The listing builds one solid part. Answer for the finished solid, in the listing's coordinates (mm). A direction names the side the tool comes from. Round coordinates to 2 decimals unless told otherwise and drop trailing zeros. Loops run counter-clockwise (first coordinate to the right, second up) from the corner with the lowest first, then second, coordinate; pieces in that order, holes last. Notation, with made-up numbers: (63, 29) - (100, 29) arc R25 ccw to (100, 62) - close; hole circle Ø4 at (14.5, -13.5). An arc over 180 degrees is marked (long way). One line per item, written item: value.
```python
from build123d import *

# Parameters (mm, degrees)
SKETCH_W        = 92
SKETCH_H        = 130
PAD_DEPTH       = 44
SKETCH001_W     = 88
SKETCH001_H     = 126
POCKET_DEPTH    = 40
SKETCH002_W     = 87.518665
SKETCH002_H     = 101
POCKET001_DEPTH = 2
SKETCH004_W     = 80
SKETCH004_H     = 80
POCKET003_DEPTH = 2
SKETCH005_W     = 88
SKETCH005_H     = 40
POCKET004_DEPTH = 2


with BuildPart() as part:
    # Sketch → Pad (new body)
    with BuildSketch(Plane.XY):
        Rectangle(SKETCH_W, SKETCH_H)
    extrude(amount=PAD_DEPTH)

    # Sketch001 → Pocket (cut)
    with BuildSketch(Plane.XY.offset(42)):
        Rectangle(SKETCH001_W, SKETCH001_H)
    extrude(amount=-POCKET_DEPTH, mode=Mode.SUBTRACT)

    # Sketch002 → Pocket001 (cut)
    with BuildSketch(Plane.XY.offset(44)):
        with Locations((0.240668, -2.5)):
            Rectangle(SKETCH002_W, SKETCH002_H)
    extrude(amount=-POCKET001_DEPTH, mode=Mode.SUBTRACT)

    # Sketch004 → Pocket003 (cut)
    with BuildSketch(Plane.XY):
        with Locations((0, -2)):
            Rectangle(SKETCH004_W, SKETCH004_H)
    extrude(amount=POCKET003_DEPTH, mode=Mode.SUBTRACT)

    # Sketch005 → Pocket004 (cut)
    with BuildSketch(Plane.XZ.offset(-65)):
        with Locations((0, 22)):
            Rectangle(SKETCH005_W, SKETCH005_H)
    extrude(amount=POCKET004_DEPTH, mode=Mode.SUBTRACT)


solid = part.part
```
1) Consider L1, parallel to X at y = -23, z = 33.5; L2, parallel to Z at x = -2.5, y = -42.5; L3, parallel to Y at x = 26.5, z = 28. Determine where each line is inside the solid, lowest interval first.
Final values:
L1: -46 to -44, 44 to 46
L2: 0 to 2
L3: -65 to -63
2) A cutting plane is placed at B-B on x = 25.5. Give the vertices of the cut face in (y, z).
Final values:
outline: (-65, 0) - (-42, 0) - (-42, 2) - (-63, 2) - (-63, 42) - (-53, 42) - (-53, 44) - (-65, 44) - close; (38, 0) - (65, 0) - (65, 2) - (38, 2) - close; (48, 42) - (65, 42) - (65, 44) - (48, 44) - close
3) This flat-tipped pin is pushed along its axis until it touches: pin 1 Ø3 at (x, z) = (26, 36.5) entering from +Y. Where does it stop, or does it pass through?
Final values:
pin 1: y = -63
4) A cutting plane is placed at A-A on y = -13.5. Give the vertices of the cut face in (x, z), and give its area (3 significant figures).
Final values:
outline: (-46, 0) - (-40, 0) - (-40, 2) - (-44, 2) - (-44, 42) - (-43.52, 42) - (-43.52, 44) - (-46, 44) - close; (40, 0) - (46, 0) - (46, 44) - (44, 44) - (44, 2) - (40, 2) - close
area: 193 mm2
5) A cutting plane is placed at C-C on z = 5. Give the vertices of the cut face in (x, y).
Final values:
outline: (-46, -65) - (46, -65) - (46, 65) - (44, 65) - (44, -63) - (-44, -63) - (-44, 65) - (-46, 65) - close
6) For faces 5 (the flat face through (-1, -65, 22)), 6 (the flat face through (-3, 44, 2)), determine the directions among +Z, -Z, +X, -X, +Y, -Y from which every point of the face is accessible in a straight line to the end or side of a thin tool.
Final values:
face 5: +Z, -Z, +X, -X, -Y
face 6: +Y
7) For a pull along Z with two mould halves and no side action, classify faces 1 (the flat face through (-44, 2, 22)), 2 (the flat face through (-3.6, 48.5, 44)), 3 (the flat face through (-46, -1, 22)), 4 (the flat face through (-1, -63, 22)) as released by +Z, released by -Z, zero draft, split by the parting line, or undercut.
Final values:
face 1: undercut
face 2: released by +Z
face 3: zero draft
face 4: undercut
